Model file for the job. Use its own axes, mm. A direction names the side the tool comes from. Give positions to 0.01 mm unless a question says otherwise; leave off trailing zeros. Loops run counter-clockwise (first coordinate to the right, second up) from the corner with the lowest first, then second, coordinate; pieces in that order, holes last. Notation, with made-up numbers: M 88,37.25 L 92,37.25 A21 cw 92,56.25 Z; hole C 64,50 d10. An arc over 180 degrees is marked long. Answer in a Markdown table with one row per item.
```python
from build123d import *

# Parameters (mm, degrees)
F0_W     = 100
F0_H     = 100
F1_DEPTH = 10
F3_DEPTH = 39.624


# Not quite as in the source:
# - a feature names something its author has since deleted; it is built from what else it names


with BuildPart() as f1:
    # F0 (on Top) → F1 (new body)
    with BuildSketch(Plane.XY):
        Rectangle(F0_W, F0_H)
    extrude(amount=-F1_DEPTH)

    # F2 (on face) → F3 (cut)
    with BuildSketch(Plane.XY):
        Polygon((10.8499823283, -18.3243404083), (20.6293614436, -5.2851692833), (18.3243404083, 10.8499823283), (5.2851692833, 20.6293614436), (-10.8499823283, 18.3243404083), (-20.6293614436, 5.2851692833), (-18.3243404083, -10.8499823283), (-5.2851692833, -20.6293614436), align=None)
    extrude(amount=-F3_DEPTH, mode=Mode.SUBTRACT)


solid = f1.part
```
Q1. Saw through at C-C (x = -3). Give the cut face in (y, z).
Reported:
| item | result |
|---|---|
| outline | M -50,-10 L -20.3,-10 L -20.3,0 L -50,0 Z; M 19.45,-10 L 50,-10 L 50,0 L 19.45,0 Z |
Q2. Saw through at A-A (z = -5). Give the cut face in (x, y), and give its area (3 significant figures).
Reported:
| item | result |
|---|---|
| outline | M -50,-50 L 50,-50 L 50,50 L -50,50 Z; hole M -20.63,5.29 L -18.32,-10.85 L -5.29,-20.63 L 10.85,-18.32 L 20.63,-5.29 L 18.32,10.85 L 5.29,20.63 L -10.85,18.32 Z |
| area | 8,720 mm² |
Q3. 3-axis set-ups, long thin cutter, end or side, ignore diameter. For faces 4 (the face through (-11.9, -15.67, -4.93)), 5 (the face through (-1, 23, -10)): which of +Z, -Z, +X, -X, +Y, -Y reach the whole face in a straight line?
Reported:
| item | result |
|---|---|
| face 4 | +Z, -Z |
| face 5 | -Z, +X, -X, +Y, -Y |
Q4. Mould opens along Y. For faces 1 (the face through (-1, 50, -5)), 2 (the face through (50, -1, -5)), 3 (the face through (-19.493, -2.669, -4.93)) say: released by +Y, released by -Y, zero draft, split by the parting line, or undercut.
Reported:
| item | result |
|---|---|
| face 1 | released by +Y |
| face 2 | zero draft |
| face 3 | undercut |
Q5. Probe probe 1 along Y at (x, z) = (-1, -9); probe 2 along X at (y, z) = (11, -2); probe 3 along Y at (x, z) = (-3, -2.25). List the from-to ranges inside material, lowest first.
Reported:
| item | result |
|---|---|
| probe 1 | -50 to -20.02, 19.73 to 50 |
| probe 2 | -50 to -16.34, 18.12 to 50 |
| probe 3 | -50 to -20.3, 19.45 to 50 |
Q6. Saw through at B-B (y = 13). Give the cut face in (x, z).
Reported:
| item | result |
|---|---|
| outline | M -50,-10 L -14.84,-10 L -14.84,0 L -50,0 Z; M 15.46,-10 L 50,-10 L 50,0 L 15.46,0 Z |
